Can you work these out from the model? Positions are in its coordinate system, mm. Face numbers are marked on the shaded views. Give positions to 0.01 mm unless a question says otherwise; leave off trailing zeros. Loops run counter-clockwise (first coordinate to the right, second up) from the corner with the lowest first, then second, coordinate; pieces in that order, holes last. Notation, with made-up numbers: (10, -27) - (68, -27) arc R19 ccw to (68, -23) - close; hole circle Ø7 at (18, 39.25). An arc over 180 degrees is marked (long way). Use a Markdown table: item, result. Add a question column.
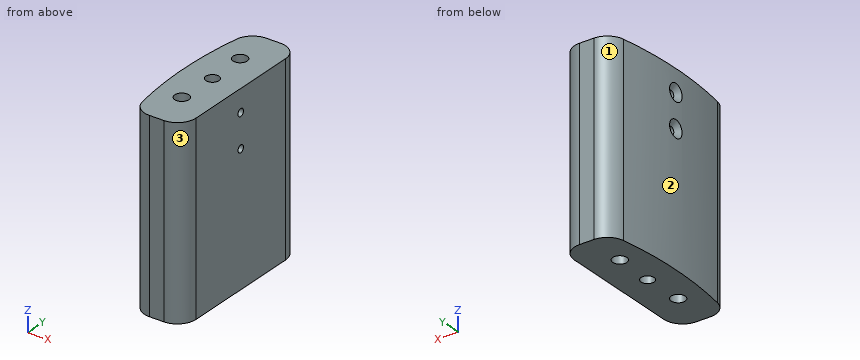
Autodesk Inventor part; units mm, degrees
ref_plane "РабПлоскость1" through (0, 0, 0) normal (0, 0, 1) x (1, 0, 0)
ref_plane "РабПлоскость2" through (-75.9237, -75.9237, 50) normal (0, 0, 1) x (0.7071, -0.7071, 0)
ref_plane "РабПлоскость3" through (-97.6153, -21.5, 25) normal (0, 0, 1) x (1, 0, 0)
ref_plane "РабПлоскость1" through (0, 0, 0) normal (0, 0, 1) x (1, 0, 0)
sketch "Эскиз1" plane through (0, 0, 0) normal (0, 0, 1) x (1, 0, 0)
  arc A0 (37.3284, -97.07) -> (37.3284, 97.07) centre (0, 0) ccw
  line L0 (-145.6, 0) -> (145.6, 0) construction
  line L1 (-101.7534, 21.5) -> (-88.7534, 21.5)
  line L2 (-88.7534, 21.5) -> (-88.7534, -21.5)
  line L3 (-88.7534, -21.5) -> (-101.7534, -21.5)
  line L4 (-101.7534, -21.5) -> (-101.7534, 21.5) construction
  line L5 (104, 0) -> (-88.7534, 0) construction
  circle A1 centre (-96.3767, 0) radius 1.75
  arc A2 (-92.7471, 47.0529) -> (-92.7471, -47.0529) centre (0, 0) ccw
  point P0 (0, 0)
  point P1 (-101.7534, 0)
  point P2 (-101.7534, 21.5)
  dimension "d0" = 43
  dimension "d1" = 13
ref_plane "РабПлоскость2" through (-75.9237, -75.9237, 50) normal (0, 0, 1) x (0.7071, -0.7071, 0)
extrude "Выдавливание1" add sketch "Эскиз1" along normal up to surface (50 mm away)
fillet "Сопряжение1" radius 5 4 edges at (-88.7534, 21.5, 25) (-88.7534, -21.5, 25) (-101.7534, -21.5, 25) (-101.7534, 21.5, 25)
sketch "Эскиз2" plane through (-88.7534, -16.5, 0) normal (1, 0, 0) x (0, 0, -1)
  line L0 (-50, 18.25) -> (-50, 14.75)
  line L1 (0, 14.75) -> (0, 18.25)
  circle A0 centre (-44, 16.5) radius 1
  line L2 (-50, 14.75) -> (0, 14.75)
  circle A1 centre (-35, 16.5) radius 1
  line L3 (-50, 16.5) -> (0, 16.5) construction
  line L4 (-50, 33) -> (-50, 0)
  point P0 (0, 16.5)
  dimension "d6" = 2
  dimension "d9" = 6
  dimension "d10" = 15
extrude "Выдавливание2" cut sketch "Эскиз2" against normal through all
chamfer "Фаска1" distance 1.3 angle 45 2 edges at (-104, 0.0084, 45) (-104, 0.0084, 36)
sketch "Эскиз3" plane through (-97.6153, -21.5, 50) normal (0, 0, 1) x (1, 0, 0)
  line L0 (0.8568, 43) -> (0.8568, 0) construction
  circle A0 centre (0.8568, 21.5) radius 1.8
  line L1 (0, 43) -> (3.8619, 43) construction
  line L2 (3.8619, 0) -> (0, 0) construction
  circle A1 centre (0.8568, 32.25) radius 1.9
  circle A2 centre (0.8568, 10.75) radius 1.9
  point P0 (97.6153, 21.5)
  point P1 (0.8568, 21.5)
  point P2 (-4.1381, 43)
  dimension "d16" = 21.5
  dimension "d17" = 10.75
  dimension "d18" = 10.75
  dimension "d19" = 3.8
extrude "Выдавливание3" cut sketch "Эскиз3" against normal blind 5.5 contours A1 | A2
ref_plane "РабПлоскость3" through (-97.6153, -21.5, 25) normal (0, 0, 1) x (1, 0, 0)
mirror "Зеркальное отражение1" about plane through (-97.6153, -21.5, 25) normal (0, 0, 1) of "Выдавливание3"
properties part number "крепление ручки"
1. Suppose I cut it at A-A (z = 10.5). List the corners of the cut face in (x, y) for me.
2. If we mould it in two halves opening along Y, with no side actions, what happens to the marked faces 1, 2 and 3? For each: released by +Y, released by -Y, zero draft, split by the parting line, or undercut.
3. Suppose I cut it at B-B (y = 0). State how many separate pieces and enclosed holes the cut face has, and give its area (3 significant figures).
4. Suppose I cut it at D-D (y = 10.75). List the corners of the cut face in (x, z) for me.
5. Suppose I cut it at C-C (x = -99.5). List the corners of the cut face in (y, z) for me, and give its area (3 significant figures).
6. Will these pins go through, and if not, where does the flat tip stop? P1, Ø1.2, axis at y = 0, z = 44, coming from the -X side; P2, Ø5, axis at y = 10.5, z = 37.5, coming from the -X side; P3, Ø1.1, axis at x = -97.5, y = -11.5, coming from the -Z side; P4, Ø10, axis at y = 15, z = 28, coming from the -X side.
7. Please list where these lines run through material, in increasing order: line 1 along Z through (x, y) = (-90.5, 0); line 2 along Y through (x, z) = (-97.75, 13); line 3 along X through (y, z) = (-0.5, 11). Write a range as [from, to].
Results below:
| question | item | result |
|---|---|---|
| 1 | outline | (-102.55, -17.33) arc R5 ccw to (-97.62, -21.5) - (-93.75, -21.5) arc R5 ccw to (-88.75, -16.5) - (-88.75, 16.5) arc R5 ccw to (-93.75, 21.5) - (-97.62, 21.5) arc R5 ccw to (-102.55, 17.33) arc R104 ccw to start; hole circle Ø3.5 at (-96.38, 0) |
| 2 | face 1 | released by +Y |
| 2 | face 2 | split by the parting line |
| 2 | face 3 | released by -Y |
| 3 | separate pieces | 6 |
| 3 | enclosed holes | 0 |
| 3 | area | 537 mm² |
| 4 | outline | (-103.44, 0) - (-98.66, 0) - (-98.66, 5.5) - (-94.86, 5.5) - (-94.86, 0) - (-88.75, 0) - (-88.75, 50) - (-94.86, 50) - (-94.86, 44.5) - (-98.66, 44.5) - (-98.66, 50) - (-103.44, 50) - close |
| 5 | outline | (-21.13, 0) - (21.13, 0) - (21.13, 50) - (-21.13, 50) - close; hole circle Ø2 at (0, 35); hole circle Ø2 at (0, 44) |
| 5 | area | 2,110 mm² |
| 6 | P1 | through |
| 6 | P2 | x = -103.69 |
| 6 | P3 | z = 5.5 |
| 6 | P4 | x = -103.52 |
| 7 | line 1 | [0, 34], [36, 43], [45, 50] |
| 7 | line 2 | [-21.5, -1.08], [1.08, 21.5] |
| 7 | line 3 | [-104, -98.05], [-94.7, -88.75] |
